from build123d import *

# Parameters (mm, degrees)
SKETCH1_R                                      = 76.2
BILLET_DEPTH                                   = 50.8
SKETCH3_R                                      = 28.575
LOX_PLATE_DEPTH                                = 17.78
SKETCH5_R                                      = 22.225
LOX_DOME_DEPTH                                 = 4.46278
SKETCH7_R                                      = 76.2
TOP_MILL_DEPTH                                 = 12.7
SKETCH12_R                                     = 60.96
KEROSENE_PLATE_DEPTH                           = 12.7
KEROSENE_INLET_3_8_NPT_TAPPED_HOLE1_AT_2_COUNT = 2
KEROSENE_INLET_3_8_NPT_TAPPED_HOLE1_AT_2_PITCH = 76.2


with BuildPart() as part:
    # Sketch1 → Billet (new body)
    with BuildSketch(Plane(origin=(0, 0, 0), x_dir=(1, 0, 0), z_dir=(0, 1, 0))):
        with Locations(Location((0, 0, 0), (0, 0, 270))):
            Circle(SKETCH1_R)
    extrude(amount=-BILLET_DEPTH)

    # Sketch3 → Lox Plate (cut)
    with BuildSketch(Plane(origin=(0, -50.8, 0), x_dir=(1, 0, 0), z_dir=(0, 1, 0))):
        with Locations(Location((0, 0, 0), (0, 0, 270))):
            Circle(SKETCH3_R)
    extrude(amount=LOX_PLATE_DEPTH, mode=Mode.SUBTRACT)

    # Sketch5 → Lox Dome (cut)
    with BuildSketch(Plane(origin=(0, -33.02, 0), x_dir=(1, 0, 0), z_dir=(0, 1, 0))):
        with Locations(Location((0, 0, 0), (0, 0, 270))):
            Circle(SKETCH5_R)
    extrude(amount=LOX_DOME_DEPTH, mode=Mode.SUBTRACT)

    # Sketch7 → Top Mill (cut)
    with BuildSketch(Plane(origin=(0, 0, 0), x_dir=(1, 0, 0), z_dir=(0, 1, 0))):
        with Locations(Location((0, 0, 0), (0, 0, 270))):
            Circle(SKETCH7_R)
    extrude(amount=-TOP_MILL_DEPTH, mode=Mode.SUBTRACT)

    # Sketch12 → Kerosene Plate (cut)
    with BuildSketch(Plane(origin=(0, -50.8, 0), x_dir=(1, 0, 0), z_dir=(0, 1, 0))):
        with Locations(Location((0, 0, 0), (0, 0, 270))):
            Circle(SKETCH12_R)
    extrude(amount=KEROSENE_PLATE_DEPTH, mode=Mode.SUBTRACT)

    # Sketch21 → Lox Inlet-1_2 NPT Tapped Hole3 (revolve, cut)
    with BuildSketch(Plane(origin=(0, -12.7, 0), x_dir=(0, 0, 1), z_dir=(1, 0, 0))):
        Polygon((0, 0), (0, 38.1), (8.9281, 38.1), (8.9281, 13.462), (10.261665792, 13.462), (10.6647361, 0), align=None)
    revolve(axis=Axis((0, -6.35, 0), (0, -1, 0)), mode=Mode.SUBTRACT)

    # Sketch25 → Kerosene Inlet-3_8 NPT Tapped Hole1 (revolve, cut)
    with BuildSketch(Plane(origin=(-38.1, -12.7, 0), x_dir=(0, 0, 1), z_dir=(1, 0, 0))):
        Polygon((0, 0), (0, 38.1), (7.1374, 38.1), (7.1374, 10.414), (8.263205494, 10.414), (8.5750146, 0), align=None)
    kerosene_inlet_3_8_npt_tapped_hole1 = revolve(axis=Axis((-38.1, -6.35, 0), (0, -1, 0)), mode=Mode.SUBTRACT)

    # Kerosene Inlet-3_8 NPT Tapped Hole1 at 2: Kerosene Inlet-3_8 NPT Tapped Hole1 ×2
    with Locations(*[(i * KEROSENE_INLET_3_8_NPT_TAPPED_HOLE1_AT_2_PITCH, 0, 0) for i in range(1, KEROSENE_INLET_3_8_NPT_TAPPED_HOLE1_AT_2_COUNT)]):
        add(kerosene_inlet_3_8_npt_tapped_hole1, mode=Mode.SUBTRACT)


solid = part.part
Could you check a few things on this model? Use its own coordinates, in mm. A direction names the side the tool comes from. Round coordinates to 2 decimals unless told otherwise and drop trailing zeros. Order: outer loops, then holes, each group sorted by start corner. A loop starts at its lowest first (then second) coordinate and runs counter-clockwise, first axis right, second up.
Q1. Imagine slicing it at D-D, the plane x = 38.1. List the corners of the cut face in (y, z) for me, then the cut area to 3 significant figures.
Geometry says:
outline: (-50.8, -65.99) - (-12.7, -65.99) - (-12.7, -8.58) - (-23.11, -8.26) - (-23.11, -7.14) - (-38.1, -7.14) - (-38.1, -47.59) - (-50.8, -47.59) - close; (-50.8, 47.59) - (-38.1, 47.59) - (-38.1, 7.14) - (-23.11, 7.14) - (-23.11, 8.26) - (-12.7, 8.58) - (-12.7, 65.99) - (-50.8, 65.99) - close
area: 3,430 mm2
Q2. Imagine slicing it at A-A, the plane x = 0. List the corners of the cut face in (y, z) for me (3 decimals), then the cut area to 3 significant figures.
Geometry says:
outline: (-50.8, -76.2) - (-12.7, -76.2) - (-12.7, -10.665) - (-26.162, -10.262) - (-26.162, -8.928) - (-28.557, -8.928) - (-28.557, -22.225) - (-33.02, -22.225) - (-33.02, -28.575) - (-38.1, -28.575) - (-38.1, -60.96) - (-50.8, -60.96) - close; (-50.8, 60.96) - (-38.1, 60.96) - (-38.1, 28.575) - (-33.02, 28.575) - (-33.02, 22.225) - (-28.557, 22.225) - (-28.557, 8.928) - (-26.162, 8.928) - (-26.162, 10.262) - (-12.7, 10.665) - (-12.7, 76.2) - (-50.8, 76.2) - close
area: 3,440 mm2
Q3. Please list where these lines run through material, in increasing order: probe 1 along X at (y, z) = (-32, 0) (3 decimals); probe 2 along X at (y, z) = (-26, 0); probe 3 along Y at (x, z) = (21.5, -47).
Geometry says:
probe 1: x = -76.2 to -45.237, -30.963 to -22.225, 22.225 to 30.963, 45.237 to 76.2
probe 2: x = -76.2 to -45.24, -30.96 to -10.27, 10.27 to 30.96, 45.24 to 76.2
probe 3: y = -38.1 to -12.7
Q4. Thinking about a two-plate mould opening in X: for faces 1 (the face through (51, -50.8, -34)), 2 (the face through (-46.367, -31.483, -60.47)), 3 (the face through (-36, -23.114, 7)), 4 (the face through (-17, -33.02, 15)), which applies, released by +X, released by -X, zero draft, split by the parting line, or undercut?
Geometry says:
face 1: zero draft
face 2: split by the parting line
face 3: undercut
face 4: undercut
Q5. Which directions (+Z, -Z, +X, -X, +Y, -Y) give clear straight access to the entire face, cutting with the end or side of a thin tool? Please do faces 5 (the face through (1.256, -35.596, -28.547)), 6 (the face through (6.368, -19.337, -8.305)), 7 (the face through (-2.682, -27.343, 8.516)).
Geometry says:
face 5: -Y
face 6: +Y
face 7: +Y, -Y
Q6. I'm going to push flat-ended pins straight in: P1, Ø17, axis at x = 3, z = 12, coming from the -Y side; P2, Ø6, axis at x = -37.5, y = -41, coming from the +Z side; P3, Ø8.5, axis at x = 38.5, z = 3.5, coming from the +Y side; P4, Ø8.5, axis at x = -38.1, z = 0, coming from the -Y side. Where does each tip first touch, or does it pass through?
Geometry says:
P1: stops at y = -28.56
P2: stops at z = 67.94
P3: stops at y = -23.11
P4: passes through
Q7. Imagine slicing it at B-B, the plane z = 0. State how many separate pieces and enclosed holes the cut face has, then the cut area to 3 significant figures.
Geometry says:
separate pieces: 4
enclosed holes: 0
area: 2,670 mm2
Q8. Imagine slicing it at C-C, the plane z = 32.5. List the corners of the cut face in (x, y) for me, then the cut area to 3 significant figures.
Geometry says:
outline: (-68.92, -50.8) - (-51.57, -50.8) - (-51.57, -38.1) - (51.57, -38.1) - (51.57, -50.8) - (68.92, -50.8) - (68.92, -12.7) - (-68.92, -12.7) - close
area: 3,940 mm2
